Read the model definition and answer for the solid it produces. Units are mm, in the model's axes. Round coordinates to 2 decimals unless told otherwise and drop trailing zeros. Write each loop counter-clockwise with the first axis right and the second up, starting at its lowest first coordinate (ties: lowest second). Pieces come first, ordered by that corner, then holes. Notation, with made-up numbers: (3.5, 2.5) - (34.5, 2.5) arc R22 cw to (34.5, 17.5) - close; hole circle Ø9 at (-30.75, 86). An arc over 180 degrees is marked (long way). Answer as CSV lines item,"result". Start each with the question number.
1) Find section D-D on x = 7.5. Determine the outline of the cut face in (y, z).
2) Consider line 1 along Y through (x, z) = (-8, 0.6); line 2 along X through (y, z) = (-3.25, 0.2); line 3 along X through (y, z) = (-4, 1.45). Determine where each line is inside the solid, lowest interval first.
3) For a pull along X with two mould halves and no side action, classify faces 1 (the cylindrical face through (-7.2, -4.1, 0.7)), 2 (the flat face through (0, 5.5, 1)), 3 (the cylindrical face through (-9.715, 5.199, 0.76)), 4 (the cylindrical face through (8.8, -4.1, 0.7)) as +X half, -X half, draft (parallel to the pull), parting line (faces both ways), or undercut.
4) Find section B-B on x = -8. Determine the outline of the cut face in (y, z).
5) Find section A-A on z = 0.9. Determine the outline of the cut face in (x, y), then the cut area to 3 significant figures.
6) Find section C-C on y = -3.5. Determine the outline of the cut face in (x, z), then the cut area to 3 significant figures.
from build123d import *

# Parameters (mm, degrees)
SZKIC1_W                       = 20
SZKIC1_H                       = 11
DODANIE_WYCI_GNI_CIE1_DEPTH    = 1.5
ZAOKR_GLENIE1_R                = 1
OTWORY_USTALAJ_CE_2_0MM1_D     = 2
OTWORY_USTALAJ_CE_2_0MM1_DEPTH = 2
OTWORY_USTALAJ_CE_2_0MM1_TIP   = 0.600860619


with BuildPart() as part:
    # Szkic1 → Dodanie-wyciągnięcie1 (new body)
    with BuildSketch(Plane.XY):
        Rectangle(SZKIC1_W, SZKIC1_H)
    extrude(amount=DODANIE_WYCI_GNI_CIE1_DEPTH)

    # Zaokrąglenie1
    zaokr_glenie1_edges = [part.edges().sort_by_distance(p)[0] for p in [
        (10, -5.5, 0.75),
        (-10, -5.5, 0.75),
        (-10, 5.5, 0.75),
        (10, 5.5, 0.75),
    ]]
    fillet(zaokr_glenie1_edges, radius=ZAOKR_GLENIE1_R)

    # Otwory ustalające Ø2.0mm1
    with Locations(Plane.XY.offset(1.5)):
        with Locations((-8, -3.5), (8, -3.5)):
            Hole(OTWORY_USTALAJ_CE_2_0MM1_D / 2, depth=OTWORY_USTALAJ_CE_2_0MM1_DEPTH)
            with Locations((0, 0, -(OTWORY_USTALAJ_CE_2_0MM1_DEPTH + OTWORY_USTALAJ_CE_2_0MM1_TIP / 2))):  # 118° drill point
                Cone(0, OTWORY_USTALAJ_CE_2_0MM1_D / 2, OTWORY_USTALAJ_CE_2_0MM1_TIP, mode=Mode.SUBTRACT)


solid = part.part
Check values:
1,outline,"(-5.5, 0) - (-4.37, 0) - (-4.37, 1.5) - (-5.5, 1.5) - close; (-2.63, 0) - (5.5, 0) - (5.5, 1.5) - (-2.63, 1.5) - close"
2,line 1,"y = -5.5 to -4.5, -2.5 to 5.5"
2,line 2,"x = -10 to -8.97, -7.03 to 7.03, 8.97 to 10"
2,line 3,"x = -10 to -8.87, -7.13 to 7.13, 8.87 to 10"
3,face 1,"undercut"
3,face 2,"draft"
3,face 3,"-X half"
3,face 4,"undercut"
4,outline,"(-5.5, 0) - (-4.5, 0) - (-4.5, 1.5) - (-5.5, 1.5) - close; (-2.5, 0) - (5.5, 0) - (5.5, 1.5) - (-2.5, 1.5) - close"
5,outline,"(-10, -4.5) arc R1 ccw to (-9, -5.5) - (9, -5.5) arc R1 ccw to (10, -4.5) - (10, 4.5) arc R1 ccw to (9, 5.5) - (-9, 5.5) arc R1 ccw to (-10, 4.5) - close; hole circle Ø2 at (-8, -3.5); hole circle Ø2 at (8, -3.5)"
5,area,"213 mm^2"
6,outline,"(-10, 0) - (-9, 0) - (-9, 1.5) - (-10, 1.5) - close; (-7, 0) - (7, 0) - (7, 1.5) - (-7, 1.5) - close; (9, 0) - (10, 0) - (10, 1.5) - (9, 1.5) - close"
6,area,"24.0 mm^2"
